from build123d import *

# Parameters (mm, degrees)
SKETCH1_W           = 78.74
SKETCH1_H           = 78.74
BOSS_EXTRUDE1_DEPTH = 4.7625
SKETCH2_R           = 4.7625
BOSS_EXTRUDE2_DEPTH = 9.525
SKETCH3_W           = 4.7752
SKETCH3_H           = 4.7752
BOSS_EXTRUDE3_DEPTH = 6.35
FILLET2_R           = 4.7625
FILLET3_R           = 0.7874
FILLET4_R           = 0.7874
FILLET5_R           = 0.7874


# Some blends are built 0.0001 mm under size
with BuildPart() as part:
    # Sketch1 → Boss-Extrude1 (new, symmetric)
    with BuildSketch(Plane.XY):
        Rectangle(SKETCH1_W, SKETCH1_H)
    extrude(amount=BOSS_EXTRUDE1_DEPTH, both=True)

    # Sketch2 → Boss-Extrude2 (add)
    with BuildSketch(Plane(origin=(39.37, 0, 0), x_dir=(0, 0, -1), z_dir=(1, 0, 0))):
        Circle(SKETCH2_R)
    boss_extrude2 = extrude(amount=BOSS_EXTRUDE2_DEPTH)

    # Sketch3 → Boss-Extrude3 (add)
    with BuildSketch(Plane(origin=(48.895, 0, 0), x_dir=(0, 0, -1), z_dir=(1, 0, 0))):
        Rectangle(SKETCH3_W, SKETCH3_H)
    boss_extrude3 = extrude(amount=BOSS_EXTRUDE3_DEPTH)

    # Mirror1: Boss-Extrude2, Boss-Extrude3 across plane
    add(boss_extrude2.mirror(Plane(origin=(0, 0, 0), x_dir=(0, 0, 1), z_dir=(1, 0, 0))))
    add(boss_extrude3.mirror(Plane(origin=(0, 0, 0), x_dir=(0, 0, 1), z_dir=(1, 0, 0))))

    # Fillet2
    fillet2_edges = [part.edges().sort_by_distance(p)[0] for p in [
        (0, -39.37, -4.7625),
        (0, -39.37, 4.7625),
        (0, 39.37, -4.7625),
        (0, 39.37, 4.7625),
    ]]
    fillet(fillet2_edges, radius=FILLET2_R - 0.0001)  # a hair under: the kernel refuses the full size

    # Fillet3
    fillet3_edges = [part.edges().sort_by_distance(p)[0] for p in [
        (-55.245, 0, -2.3876),
        (-55.245, -2.3876, 0),
        (-55.245, 0, 2.3876),
        (-55.245, 2.3876, 0),
    ]]
    fillet(fillet3_edges, radius=FILLET3_R)

    # Fillet4
    fillet4_edges = [part.edges().sort_by_distance(p)[0] for p in [
        (55.245, 0, -2.3876),
        (55.245, 2.3876, 0),
        (55.245, 0, 2.3876),
        (55.245, -2.3876, 0),
    ]]
    fillet(fillet4_edges, radius=FILLET4_R)

    # Fillet5
    # the kernel refuses this fillet: 0.7874 mm, written as the material it takes off along each edge
    with BuildSketch(Plane(origin=(54.4576, -1.6002, -1.6002), x_dir=(0, 0, -1), z_dir=(0, -1, 0))) as fillet5_piece_1_section:
        Polygon((0, 0), (FILLET5_R, 0), (FILLET5_R, FILLET5_R), (0, FILLET5_R), align=None)
    fillet5_piece_1 = extrude(amount=FILLET5_R, mode=Mode.PRIVATE)
    fillet5_piece_1 = fillet5_piece_1 - Plane(origin=(54.4576, -1.6002, -1.6002), x_dir=(-0.7071067811865475, 0, 0.7071067811865475), z_dir=(0, -1, 0)) * Sphere(FILLET5_R, mode=Mode.PRIVATE)
    add(fillet5_piece_1, mode=Mode.SUBTRACT)
    with BuildSketch(Plane(origin=(54.4576, -1.6002, 1.6002), x_dir=(0, 0, 1), z_dir=(0, -1, 0))) as fillet5_piece_2_section:
        Polygon((0, 0), (FILLET5_R, 0), (FILLET5_R, -FILLET5_R), (0, -FILLET5_R), align=None)
    fillet5_piece_2 = extrude(amount=FILLET5_R, mode=Mode.PRIVATE)
    fillet5_piece_2 = fillet5_piece_2 - Plane(origin=(54.4576, -1.6002, 1.6002), x_dir=(-0.7071067811865475, 0, -0.7071067811865475), z_dir=(0, -1, 0)) * Sphere(FILLET5_R, mode=Mode.PRIVATE)
    add(fillet5_piece_2, mode=Mode.SUBTRACT)
    with BuildSketch(Plane(origin=(54.4576, 1.6002, -1.6002), x_dir=(0, 1, 0), z_dir=(0, 0, -1))) as fillet5_piece_3_section:
        Polygon((0, 0), (FILLET5_R, 0), (FILLET5_R, FILLET5_R), (0, FILLET5_R), align=None)
    fillet5_piece_3 = extrude(amount=FILLET5_R, mode=Mode.PRIVATE)
    fillet5_piece_3 = fillet5_piece_3 - Plane(origin=(54.4576, 1.6002, -1.6002), x_dir=(-0.7071067811865475, -0.7071067811865475, 0), z_dir=(0, 0, -1)) * Sphere(FILLET5_R, mode=Mode.PRIVATE)
    add(fillet5_piece_3, mode=Mode.SUBTRACT)
    with BuildSketch(Plane(origin=(54.4576, 1.6002, 1.6002), x_dir=(0, 1, 0), z_dir=(0, 0, 1))) as fillet5_piece_4_section:
        Polygon((0, 0), (FILLET5_R, 0), (FILLET5_R, -FILLET5_R), (0, -FILLET5_R), align=None)
    fillet5_piece_4 = extrude(amount=FILLET5_R, mode=Mode.PRIVATE)
    fillet5_piece_4 = fillet5_piece_4 - Plane(origin=(54.4576, 1.6002, 1.6002), x_dir=(-0.7071067811865475, -0.7071067811865475, 0), z_dir=(0, 0, 1)) * Sphere(FILLET5_R, mode=Mode.PRIVATE)
    add(fillet5_piece_4, mode=Mode.SUBTRACT)
    with BuildSketch(Plane(origin=(-54.4576, 1.6002, 1.6002), x_dir=(0, 0, 1), z_dir=(0, 1, 0))) as fillet5_piece_5_section:
        Polygon((0, 0), (FILLET5_R, 0), (FILLET5_R, -FILLET5_R), (0, -FILLET5_R), align=None)
    fillet5_piece_5 = extrude(amount=FILLET5_R, mode=Mode.PRIVATE)
    fillet5_piece_5 = fillet5_piece_5 - Plane(origin=(-54.4576, 1.6002, 1.6002), x_dir=(0.7071067811865475, 0, -0.7071067811865475), z_dir=(0, 1, 0)) * Sphere(FILLET5_R, mode=Mode.PRIVATE)
    add(fillet5_piece_5, mode=Mode.SUBTRACT)
    with BuildSketch(Plane(origin=(-54.4576, 1.6002, -1.6002), x_dir=(0, 1, 0), z_dir=(0, 0, -1))) as fillet5_piece_6_section:
        Polygon((0, 0), (FILLET5_R, 0), (FILLET5_R, -FILLET5_R), (0, -FILLET5_R), align=None)
    fillet5_piece_6 = extrude(amount=FILLET5_R, mode=Mode.PRIVATE)
    fillet5_piece_6 = fillet5_piece_6 - Plane(origin=(-54.4576, 1.6002, -1.6002), x_dir=(0.7071067811865475, -0.7071067811865475, 0), z_dir=(0, 0, -1)) * Sphere(FILLET5_R, mode=Mode.PRIVATE)
    add(fillet5_piece_6, mode=Mode.SUBTRACT)
    with BuildSketch(Plane(origin=(-54.4576, -1.6002, 1.6002), x_dir=(0, 0, 1), z_dir=(0, -1, 0))) as fillet5_piece_7_section:
        Polygon((0, 0), (FILLET5_R, 0), (FILLET5_R, FILLET5_R), (0, FILLET5_R), align=None)
    fillet5_piece_7 = extrude(amount=FILLET5_R, mode=Mode.PRIVATE)
    fillet5_piece_7 = fillet5_piece_7 - Plane(origin=(-54.4576, -1.6002, 1.6002), x_dir=(0.7071067811865475, 0, -0.7071067811865475), z_dir=(0, -1, 0)) * Sphere(FILLET5_R, mode=Mode.PRIVATE)
    add(fillet5_piece_7, mode=Mode.SUBTRACT)
    with BuildSketch(Plane(origin=(-54.4576, -1.6002, -1.6002), x_dir=(0, 0, -1), z_dir=(0, -1, 0))) as fillet5_piece_8_section:
        Polygon((0, 0), (FILLET5_R, 0), (FILLET5_R, -FILLET5_R), (0, -FILLET5_R), align=None)
    fillet5_piece_8 = extrude(amount=FILLET5_R, mode=Mode.PRIVATE)
    fillet5_piece_8 = fillet5_piece_8 - Plane(origin=(-54.4576, -1.6002, -1.6002), x_dir=(0.7071067811865475, 0, 0.7071067811865475), z_dir=(0, -1, 0)) * Sphere(FILLET5_R, mode=Mode.PRIVATE)
    add(fillet5_piece_8, mode=Mode.SUBTRACT)
    with BuildSketch(Plane(origin=(48.895, -2.3876, -2.3876), x_dir=(0, 0, 1), z_dir=(1, 0, 0)), Plane(origin=(-48.895, -2.3876, 2.3876), x_dir=(0, 0, -1), z_dir=(-1, 0, 0)), Plane(origin=(48.895, 2.3876, -2.3876), x_dir=(0, -1, 0), z_dir=(1, 0, 0))) as fillet5_piece_9:
        with BuildLine():
            CenterArc((FILLET5_R, -FILLET5_R), FILLET5_R, 90, 90)
            Line((0, -FILLET5_R), (0, 0))
            Line((0, 0), (FILLET5_R, 0))
        make_face()
    extrude(amount=5.5626, mode=Mode.SUBTRACT)
    with BuildSketch(Plane(origin=(-48.895, -2.3876, -2.3876), x_dir=(0, 0, 1), z_dir=(-1, 0, 0)), Plane(origin=(-48.895, 2.3876, -2.3876), x_dir=(0, -1, 0), z_dir=(-1, 0, 0)), Plane(origin=(-48.895, 2.3876, 2.3876), x_dir=(0, 0, -1), z_dir=(-1, 0, 0)), Plane(origin=(48.895, 2.3876, 2.3876), x_dir=(0, -1, 0), z_dir=(1, 0, 0)), Plane(origin=(48.895, -2.3876, 2.3876), x_dir=(0, 0, -1), z_dir=(1, 0, 0))) as fillet5_piece_10:
        with BuildLine():
            CenterArc((FILLET5_R, FILLET5_R), FILLET5_R, 180, 90)
            Line((0, FILLET5_R), (0, 0))
            Line((0, 0), (FILLET5_R, 0))
        make_face()
    extrude(amount=5.5626, mode=Mode.SUBTRACT)


solid = part.part
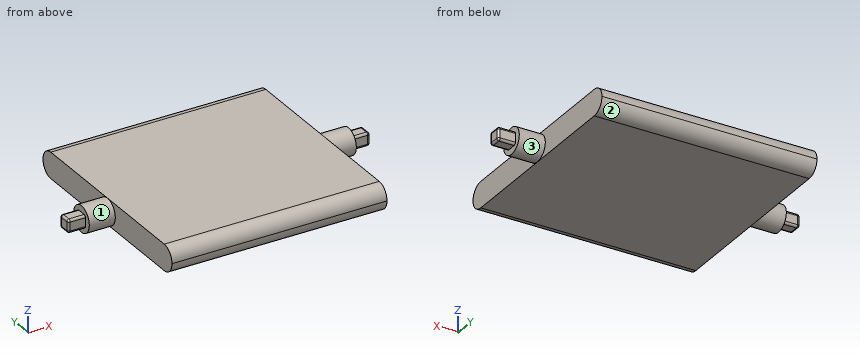
Verification items for the finished model (mm, model axes). Face numbers are marked on the shaded views. A direction names the side the tool comes from. Give positions to 0.01 mm unless a question says otherwise; leave off trailing zeros. Write each loop counter-clockwise with the first axis right and the second up, starting at its lowest first coordinate (ties: lowest second). Pieces come first, ordered by that corner, then holes. Notation, with made-up numbers: M 23,22.5 L 44,22.5 A19 ccw 44,49.5 Z; hole C 34,78.5 d7. An arc over 180 degrees is marked long. Use CSV: the item, a comma, the result in double quotes.
1) Go/stop test with flat-tipped pins: pin 1 Ø3.5 at (x, y) = (50.5, -1) entering from -Z; pin 2 Ø3 at (y, z) = (13.5, 0) entering from +X; pin 3 Ø1 at (x, z) = (-52.5, 0) entering from +Y. Record where each tip stops, or that it passes through.
Final values:
pin 1,"z = -4.75"
pin 2,"x = 39.37"
pin 3,"y = 2.39"
2) Material ranges on line 1 along X through (y, z) = (-27.5, -2.75); line 2 along X through (y, z) = (-1, -3) (3 decimals); line 3 along Y through (x, z) = (-4, -0.75), recorded low to high.
Final values:
line 1,"-39.37 to 39.37"
line 2,"-48.895 to 48.895"
line 3,"-39.31 to 39.31"
3) Access from +Z, -Z, +X, -X, +Y, -Y to the whole of each face (thin tool, end or side, straight path). Record for the marked faces 1, 2 and 3.
Final values:
face 1,"-X"
face 2,"-Z, +X, -X, +Y"
face 3,"+X"
4) Cross-section at B-B (y = -29.5). Enter the section's corners in (x, z).
Final values:
outline,"M -39.37,-4.76 L 39.37,-4.76 L 39.37,4.76 L -39.37,4.76 Z"
